The model under review builds one solid part; all positions refer to its coordinate system, in mm. Face numbers are marked on the shaded views. A direction names the side the tool comes from. Round coordinates to 2 decimals unless told otherwise and drop trailing zeros. Write each loop counter-clockwise with the first axis right and the second up, starting at its lowest first coordinate (ties: lowest second). Pieces come first, ordered by that corner, then holes. Notation, with made-up numbers: M 10,-2 L 23,-2 A15 cw 23,13 Z; hole C 75.25,33.5 d1. An arc over 180 degrees is marked long. One line per item, written item: value. Start each with the question number.
1) For P1, Ø0.7, axis at x = 0, z = -1.5, coming from the +Y side; P2, Ø5, axis at x = -2, y = -5, coming from the -Z side; P3, Ø0.5, axis at y = -18, z = -1, coming from the +X side; P4, Ø3, axis at x = 0, y = 0, coming from the +Z side, all flat-tipped, find the tip position at first contact; note any pin that passes through.
2) Wall thickness on probe 1 along Y at (x, z) = (0, 0.4); probe 2 along X at (y, z) = (0, 0.9); probe 3 along Y at (x, z) = (3, 0.75): over which ranges is each line inside the solid? List them lowest first.
3) Take a section at D-D, the plane y = -13.5. Write out the cut boundary in (x, z).
4) Take a section at B-B, the plane x = 0. Write out the cut boundary in (y, z), and give its area (3 significant figures).
5) Mouldability with a two-part tool opening along Y and no side actions: class the marked faces 1, 2, 3 and 4 as +Y half, -Y half, draft (parallel to the pull), parting line (faces both ways), or undercut.
6) Take a section at A-A, the plane y = 0. Write out the cut boundary in (x, z), and give its area (3 significant figures).
7) Tool access review of the marked faces 5, 6, 7 and 8: name each direction out of +Z, -Z, +X, -X, +Y, -Y from which nothing blocks a thin tool from reaching the whole face with its end or side.
8) Take a section at C-C, the plane z = -1.25. Write out the cut boundary in (x, y), and give its area (3 significant figures).
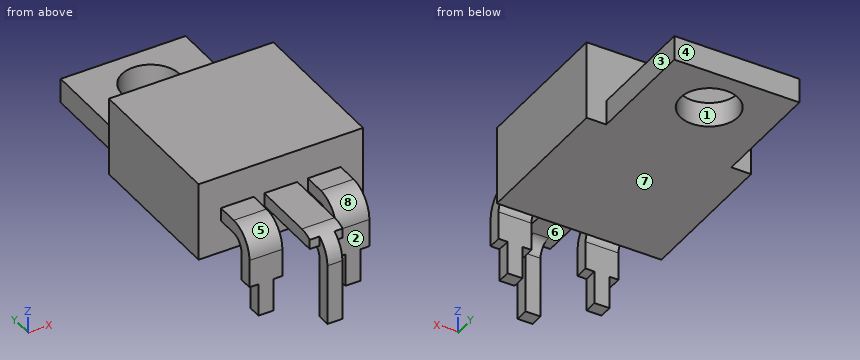
from build123d import *

# Parameters (mm, degrees)
SKETCH_1_R                  = 1.75
EXTRUDE_1_DEPTH             = 4.8
SKETCH_2_W                  = 12.314395844
SKETCH_2_H                  = 6.906876711
CUT_EXTRUDE_1_DEPTH         = 3.3
SKETCH_3_W                  = 2
SKETCH_3_H                  = 0.8
EXTRUDE_2_DEPTH             = 5
SKETCH_4_W                  = 2
SKETCH_4_H                  = 0.8
CUT_EXTRUDE_2_DEPTH         = 2.5
SKETCH_5_W                  = 0.911290814
SKETCH_5_H                  = 0.8
SKETCH_5_W_2                = 2
EXTRUDE_3_DEPTH             = 2.5
EXTRUDE_3_DIRECTION_2_REACH = 21.081
SKETCH_6_W                  = 0.493961758
SKETCH_6_H                  = 0.8
SKETCH_6_W_2                = 0.594747428
CUT_EXTRUDE_3_DEPTH         = 0.4
FILLET_1_R                  = 0.8
FILLET_2_R                  = 1.6
SKETCH_7_W                  = 0.911290814
SKETCH_7_H                  = 0.8
SKETCH_7_W_2                = 0.911290815
EXTRUDE_4_DEPTH             = 2


with BuildPart() as part:
    # Эскиз1 → Вытянуть1 (new body)
    with BuildSketch(Plane.XY):
        Polygon((-3.8, 2.8), (-3.8, -4.1), (-5, -4.1), (-5, -13.2), (5, -13.2), (5, -4.1), (3.8, -4.1), (3.8, 2.8), align=None)
        Circle(SKETCH_1_R, mode=Mode.SUBTRACT)
    extrude(amount=EXTRUDE_1_DEPTH)

    # Эскиз2 → Вырез-Вытянуть1 (cut)
    with BuildSketch(Plane.XY.offset(4.8)):
        with Locations((-0.012289816, -0.646561645)):
            Rectangle(SKETCH_2_W, SKETCH_2_H)
    extrude(amount=-CUT_EXTRUDE_1_DEPTH, mode=Mode.SUBTRACT)

    # Эскиз3 → Вытянуть2 (add)
    with BuildSketch(Plane.XZ.offset(13.2)):
        with Locations((0, 2.4)):
            Rectangle(SKETCH_3_W, SKETCH_3_H)
        with Locations((-2.644349478, 2.4)):
            Rectangle(SKETCH_3_W, SKETCH_3_H)
        with Locations((2.644349478, 2.4)):
            Rectangle(SKETCH_3_W, SKETCH_3_H)
    extrude(amount=EXTRUDE_2_DEPTH)

    # Эскиз4 → Вырез-Вытянуть2 (cut)
    with BuildSketch(Plane.XZ.offset(18.2)):
        with Locations((2.644349478, 2.4)):
            Rectangle(SKETCH_4_W, SKETCH_4_H)
        with Locations((-2.644349478, 2.4)):
            Rectangle(SKETCH_4_W, SKETCH_4_H)
    extrude(amount=-CUT_EXTRUDE_2_DEPTH, mode=Mode.SUBTRACT)

    # Эскиз5 → Вытянуть3 (add)
    with BuildSketch(Plane(origin=(0, 0, 2), x_dir=(-1, 0, 0), z_dir=(0, 0, -1))):
        with Locations((-0.050392835, -18.2)):
            Rectangle(SKETCH_5_W, SKETCH_5_H)
        with Locations((2.644349478, -15.7)):
            Rectangle(SKETCH_5_W_2, SKETCH_5_H)
        with Locations((-2.644349478, -15.7)):
            Rectangle(SKETCH_5_W_2, SKETCH_5_H)
    extrude(amount=EXTRUDE_3_DEPTH)

    # Вытянуть3 direction 2: up to this face of the body (flat: up to its plane)
    extrude_3_direction_2_end = Plane(part.part.faces().sort_by_distance((-2.644349478, -14.45, 2.8))[0])
    # Эскиз5 → Вытянуть3 direction 2 (add, up to the picked face)
    with BuildSketch(Plane(origin=(0, 0, 2), x_dir=(-1, 0, 0), z_dir=(0, 0, -1)), mode=Mode.PRIVATE) as extrude_3_direction_2_sk1:
        with Locations((-0.050392835, -18.2)):
            Rectangle(SKETCH_5_W, SKETCH_5_H)
    extrude_3_direction_2_tool1 = split(extrude(extrude_3_direction_2_sk1.sketch, amount=-EXTRUDE_3_DIRECTION_2_REACH, mode=Mode.PRIVATE), bisect_by=extrude_3_direction_2_end, keep=Keep.BOTH, mode=Mode.PRIVATE)
    # Эскиз5 → Вытянуть3 direction 2 (add, up to the picked face)
    with BuildSketch(Plane(origin=(0, 0, 2), x_dir=(-1, 0, 0), z_dir=(0, 0, -1)), mode=Mode.PRIVATE) as extrude_3_direction_2_sk2:
        with Locations((2.644349478, -15.7)):
            Rectangle(SKETCH_5_W_2, SKETCH_5_H)
    extrude_3_direction_2_tool2 = split(extrude(extrude_3_direction_2_sk2.sketch, amount=-EXTRUDE_3_DIRECTION_2_REACH, mode=Mode.PRIVATE), bisect_by=extrude_3_direction_2_end, keep=Keep.BOTH, mode=Mode.PRIVATE)
    # Эскиз5 → Вытянуть3 direction 2 (add, up to the picked face)
    with BuildSketch(Plane(origin=(0, 0, 2), x_dir=(-1, 0, 0), z_dir=(0, 0, -1)), mode=Mode.PRIVATE) as extrude_3_direction_2_sk3:
        with Locations((-2.644349478, -15.7)):
            Rectangle(SKETCH_5_W_2, SKETCH_5_H)
    extrude_3_direction_2_tool3 = split(extrude(extrude_3_direction_2_sk3.sketch, amount=-EXTRUDE_3_DIRECTION_2_REACH, mode=Mode.PRIVATE), bisect_by=extrude_3_direction_2_end, keep=Keep.BOTH, mode=Mode.PRIVATE)
    add(extrude_3_direction_2_tool1.solids().sort_by(Axis((0.050393, -18.2, 2), (0, 0, 1)))[0])
    add(extrude_3_direction_2_tool2.solids().sort_by(Axis((-2.644349, -15.7, 2), (0, 0, 1)))[0])
    add(extrude_3_direction_2_tool3.solids().sort_by(Axis((2.644349, -15.7, 2), (0, 0, 1)))[0])

    # Эскиз6 → Вырез-Вытянуть3 (cut)
    with BuildSketch(Plane.XZ.offset(18.2)):
        with Locations((0.753019121, 2.4)):
            Rectangle(SKETCH_6_W, SKETCH_6_H)
        with Locations((-0.702626286, 2.4)):
            Rectangle(SKETCH_6_W_2, SKETCH_6_H)
    extrude(amount=-CUT_EXTRUDE_3_DEPTH, mode=Mode.SUBTRACT)

    # Скругление1
    fillet_1_edges = [part.edges().sort_by_distance(p)[0] for p in [
        (0.050392835, -17.8, 2),
        (-2.644349478, -15.3, 2),
        (2.644349478, -15.3, 2),
    ]]
    fillet(fillet_1_edges, radius=FILLET_1_R)

    # Скругление2
    fillet_2_edges = [part.edges().sort_by_distance(p)[0] for p in [
        (-2.644349478, -16.1, 2.8),
        (0.050392835, -18.6, 2.8),
        (2.644349478, -16.1, 2.8),
    ]]
    fillet(fillet_2_edges, radius=FILLET_2_R)

    # Эскиз7 → Вытянуть4 (add)
    with BuildSketch(Plane(origin=(0, 0, -0.5), x_dir=(-1, 0, 0), z_dir=(0, 0, -1))):
        with Locations((-0.050392835, -18.2)):
            Rectangle(SKETCH_7_W, SKETCH_7_H)
        with Locations((-2.644349478, -15.7)):
            Rectangle(SKETCH_7_W_2, SKETCH_7_H)
        with Locations((2.644349478, -15.7)):
            Rectangle(SKETCH_7_W_2, SKETCH_7_H)
    extrude(amount=EXTRUDE_4_DEPTH)


solid = part.part
Checked values:
1. P1: stops at y = -17.8
1. P2: stops at z = 0
1. P3: stops at x = 0.51
1. P4: passes through
2. probe 1: y = -18.6 to -17.8, -13.2 to -1.75, 1.75 to 2.8
2. probe 2: x = -3.8 to -1.75, 1.75 to 3.8
2. probe 3: y = -16.1 to -15.3, -13.2 to 2.8
3. outline: M -3.64,2 L -1.64,2 L -1.64,2.8 L -3.64,2.8 Z; M -1,2 L 1,2 L 1,2.8 L -1,2.8 Z; M 1.64,2 L 3.64,2 L 3.64,2.8 L 1.64,2.8 Z
4. outline: M -18.6,-2.5 L -17.8,-2.5 L -17.8,1.2 A0.8 cw -17,2 L -13.2,2 L -13.2,0 L -1.75,0 L -1.75,1.5 L -4.1,1.5 L -4.1,4.8 L -13.2,4.8 L -13.2,2.8 L -17,2.8 A1.6 ccw -18.6,1.2 Z; M 1.75,0 L 2.8,0 L 2.8,1.5 L 1.75,1.5 Z
4. area: 56.3 mm2
5. face 1: undercut
5. face 2: -Y half
5. face 3: draft
5. face 4: +Y half
6. outline: M -3.8,0 L -1.75,0 L -1.75,1.5 L -3.8,1.5 Z; M 1.75,0 L 3.8,0 L 3.8,1.5 L 1.75,1.5 Z
6. area: 6.15 mm2
7. face 5: +Z, -X, -Y
7. face 6: -Z
7. face 7: -Z, +X, -X, +Y
7. face 8: +Z, +X, -Y
8. outline: M -3.1,-16.1 L -2.19,-16.1 L -2.19,-15.3 L -3.1,-15.3 Z; M -0.41,-18.6 L 0.51,-18.6 L 0.51,-17.8 L -0.41,-17.8 Z; M 2.19,-16.1 L 3.1,-16.1 L 3.1,-15.3 L 2.19,-15.3 Z
8. area: 2.19 mm2
